from build123d import *

# Parameters (mm, degrees)
F0_R     = 20
F0_R_2   = 15.5
F1_DEPTH = 2
F2_R     = 15.5
F2_R_2   = 14.75
F3_DEPTH = 3.2
F4_R     = 1


with BuildPart() as f1:
    # F0 (on Top) → F1 (new body)
    with BuildSketch(Plane.XY):
        Circle(F0_R)
        Circle(F0_R_2, mode=Mode.SUBTRACT)
    extrude(amount=F1_DEPTH)

    # F2 (on Top) → F3 (join)
    with BuildSketch(Plane.XY):
        Circle(F2_R)
        Circle(F2_R_2, mode=Mode.SUBTRACT)
    extrude(amount=F3_DEPTH)

    # F4
    f4_edges = [f1.edges().sort_by_distance(p)[0] for p in [
        (-20, 0, 0),
        (-14.75, 0, 0),
    ]]
    fillet(f4_edges, radius=F4_R)


solid = f1.part
Check sheet for the modelled part. Datum: model origin and axes. Units: mm. A direction names the side the tool comes from. Give positions to 0.01 mm unless a question says otherwise; leave off trailing zeros. Loops run counter-clockwise (first coordinate to the right, second up) from the corner with the lowest first, then second, coordinate; pieces in that order, holes last. Notation, with made-up numbers: M -15,50 L 3,50 A27 cw 3,66 Z; hole C 23,31 d2. An arc over 180 degrees is marked long. Return JSON: item names as keys, results as strings. Group by question number.
1. Tool access check on faces 4 (the flat face through (14, -6, 3.2)), 5 (the flat face through (10.3, -11.8, 2)). Record the directions out of +Z, -Z, +X, -X, +Y, -Y that give a thin tool (end or side, any length) a straight path to the whole face; none if there is none.
2. Mould release check, pull along X, two halves, no side actions. Record for faces 1 (the flat face through (3, 16, 0)), 2 (the cylindrical face through (-4.336, -19.524, 1.493)), 3 (the cylindrical face through (14.07, 4.43, 2.08)): released by +X, released by -X, zero draft, split by the parting line, or undercut.
3. Go/stop test with flat-tipped pins: pin 1 (1.5 mm diameter, centred on x = -12.5, y = -12, fed in from +Z); pin 2 (1 mm diameter, centred on x = 12, y = -16, fed in from -Z). Record where each tip stops, or that it passes through.
4. Thickness scan on L1, parallel to Y at x = 0, z = 2.2; L2, parallel to Z at x = -15.5, y = 3; L3, parallel to X at y = 11, z = 2.9. Record the ranges inside material, lowest first.
5. Cross-section at A-A on x = 0. Record the boundary of the cut face in (y, z), plus the area to 3 significant figures.
Return value:
{
 "1": {"face 4": "+Z, +X, -X, +Y, -Y", "face 5": "+Z"},
 "2": {"face 1": "zero draft", "face 2": "split by the parting line", "face 3": "undercut"},
 "3": {"pin 1": "z = 2", "pin 2": "z = 0.13"},
 "4": {"L1": "-15.5 to -14.75, 14.75 to 15.5", "L2": "0 to 2", "L3": "-10.92 to -9.83, 9.83 to 10.92"},
 "5": {"outline": "M -20,1 A1 ccw -19,0 L -15.75,0 A1 ccw -14.75,1 L -14.75,3.2 L -15.5,3.2 L -15.5,2 L -20,2 Z; M 14.75,1 A1 ccw 15.75,0 L 19,0 A1 ccw 20,1 L 20,2 L 15.5,2 L 15.5,3.2 L 14.75,3.2 Z", "area": "21.9 mm^2"}
}
